```python
from build123d import *

# Parameters (mm, degrees)
SKETCH_1_W             = 14
SKETCH_1_H             = 10
EXTRUDE_1_DEPTH        = 10
SKETCH_2_R             = 1
CUT_EXTRUDE_1_DEPTH    = 10
SKETCH_3_W             = 14
SKETCH_3_H             = 4.2
CUT_EXTRUDE_2_DEPTH    = 10
FILLET_1_R             = 1
CUT_EXTRUDE_START      = -10
CUT_EXTRUDE_3_DEPTH    = 38.71788575
PATTERN_LINEAR_1_COUNT = 7
PATTERN_LINEAR_1_PITCH = 2.4
FILLET_2_R             = 1


with BuildPart() as part:
    # 草图1 → 凸台-拉伸1 (new body)
    with BuildSketch(Plane.XY):
        Rectangle(SKETCH_1_W, SKETCH_1_H)
        Polygon((-11, -5), (-7, -5), (7, -5), (-11, -25), align=None)
    extrude(amount=EXTRUDE_1_DEPTH)

    # 草图2 → 切除-拉伸1 (cut)
    with BuildSketch(Plane.XY.offset(10)):
        with Locations((-5, 3)):
            Circle(SKETCH_2_R)
        with Locations((5, 3)):
            Circle(SKETCH_2_R)
    extrude(amount=-CUT_EXTRUDE_1_DEPTH, mode=Mode.SUBTRACT)

    # 草图3 → 切除-拉伸2 (cut)
    with BuildSketch(Plane(origin=(0, 5, 0), x_dir=(1, 0, 0), z_dir=(0, 1, 0))):
        with Locations((0, -4.9)):
            Rectangle(SKETCH_3_W, SKETCH_3_H)
    extrude(amount=-CUT_EXTRUDE_2_DEPTH, mode=Mode.SUBTRACT)

    # 圆角1
    fillet_1_edges = [part.edges().sort_by_distance(p)[0] for p in [
        (-11, -25, 5),
        (-11, -5, 5),
    ]]
    fillet(fillet_1_edges, radius=FILLET_1_R)

    # 草图5 → 切除-拉伸3 (cut)
    with BuildSketch(Plane.XY.offset(10).offset(CUT_EXTRUDE_START)):
        Polygon((-75.789683565, -61.267851911), (-11, -22.394041773), (-10.5, -22.094041773), (-10.5, -21.494041773), (-11, -21.194041773), (-75.789683565, 17.679768366), (-226.903894824, 17.679768366), (-226.903894824, -61.267851911), align=None)
    cut_extrude_3 = extrude(amount=CUT_EXTRUDE_3_DEPTH, mode=Mode.SUBTRACT)

    # 阵列(线性)1: 切除-拉伸3 ×7
    with Locations(*[(0, i * PATTERN_LINEAR_1_PITCH, 0) for i in range(1, PATTERN_LINEAR_1_COUNT)]):
        add(cut_extrude_3, mode=Mode.SUBTRACT)

    # 圆角2
    fillet_2_edges = [part.edges().sort_by_distance(p)[0] for p in [
        (-7, 5, 8.5),
        (7, 5, 8.5),
        (-7, 5, 1.4),
        (7, 5, 1.4),
    ]]
    fillet(fillet_2_edges, radius=FILLET_2_R)


solid = part.part
```
Could you check a few things on this model? Use its own coordinates, in mm. A direction names the side the tool comes from. Coordinates: 2 decimals unless noted, no trailing zeros. Loops run counter-clockwise (first coordinate to the right, second up) from the corner with the lowest first, then second, coordinate; pieces in that order, holes last.
1) Will these pins go through, and if not, where does the flat tip stop? pin 1 Ø1.5 at (x, z) = (-3, 2.5) entering from -Y; pin 2 Ø0.7 at (y, z) = (-14.5, 5.5) entering from -X; pin 3 Ø0.8 at (y, z) = (-1, 1) entering from -X.
Reported:
pin 1: stops at y = -16.94
pin 2: stops at x = -10.74
pin 3: stops at x = -7
2) Imagine slicing it at B-B (x = 5). List the corners of the cut face in (y, z) for me.
Reported:
outline: (-7.22, 0) - (2, 0) - (2, 2.8) - (-5, 2.8) - (-5, 7) - (2, 7) - (2, 10) - (-7.22, 10) - close; (4, 0) - (5, 0) - (5, 2.8) - (4, 2.8) - close; (4, 7) - (5, 7) - (5, 10) - (4, 10) - close
3) Which directions (+Z, -Z, +X, -X, +Y, -Y) give clear straight access to the entire face, cutting with the end or side of a thin tool? Please do faces 4 (the face through (-7, -1, 8)), 5 (the face through (0, 0, 2.8)), 6 (the face through (-4, -5, 5)).
Reported:
face 4: +Z, -Z, -X, +Y
face 5: +X, -X, +Y
face 6: -X, +Y
4) Please list where these lines run through material, in increasing order: line 1 along Z through (x, y) = (6, -4.75); line 2 along Y through (x, z) = (-5, 8.25); line 3 along X through (y, z) = (0.5, 7.25).
Reported:
line 1: z = 0 to 2.8, 7 to 10
line 2: y = -18.33 to 2, 4 to 5
line 3: x = -7 to 7
5) Thinking about a two-plate mould opening in X: for faces 1 (the face through (-5.737, 3.676, 1.42)), 2 (the face through (0, 5, 1)), 3 (the face through (7, -1, 1)), which applies, released by +X, released by -X, zero draft, split by the parting line, or undercut?
Reported:
face 1: undercut
face 2: zero draft
face 3: released by +X
6) Imagine slicing it at D-D (x = -2.25). List the corners of the cut face in (y, z) for me, and give its area (3 significant figures).
Reported:
outline: (-15.28, 0) - (5, 0) - (5, 2.8) - (-5, 2.8) - (-5, 7) - (5, 7) - (5, 10) - (-15.28, 10) - close
area: 161 mm2
7) Imagine slicing it at C-C (z = 8.5). State how many separate pieces and enclosed holes the cut face has, and give its area (3 significant figures).
Reported:
separate pieces: 1
enclosed holes: 2
area: 309 mm2
8) Imagine slicing it at A-A (y = 3). List the corners of the cut face in (x, z) for me.
Reported:
outline: (-7, 0) - (-6, 0) - (-6, 2.8) - (-7, 2.8) - close; (-7, 7) - (-6, 7) - (-6, 10) - (-7, 10) - close; (-4, 0) - (4, 0) - (4, 2.8) - (-4, 2.8) - close; (-4, 7) - (4, 7) - (4, 10) - (-4, 10) - close; (6, 0) - (7, 0) - (7, 2.8) - (6, 2.8) - close; (6, 7) - (7, 7) - (7, 10) - (6, 10) - close
